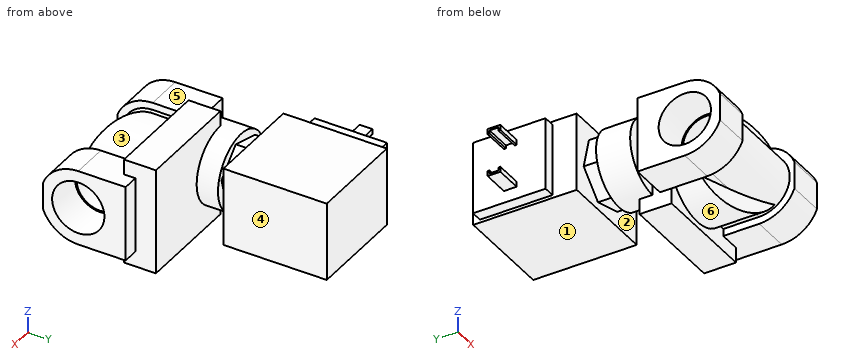
```python
from build123d import *

# Parameters (mm, degrees)
SKETCH1_R                = 18.0086
BOSS_EXTRUDE1_DEPTH      = 20.9296
CUT_EXTRUDE1_DEPTH       = 19.0086
CUT_EXTRUDE1_DEPTH_BACK  = 19.0086
BOSS_EXTRUDE2_DEPTH      = 16.129
BOSS_EXTRUDE3_DEPTH      = 14.0335
SKETCH6_W                = 40.132
SKETCH6_H                = 40.132
BOSS_EXTRUDE4_DEPTH      = 12.0777
SKETCH7_R                = 14.2875
BOSS_EXTRUDE5_DEPTH      = 8.0772
BOSS_EXTRUDE5_DEPTH_BACK = 4.826
BOSS_EXTRUDE6_DEPTH      = 5.9817
SKETCH11_W               = 41.656
SKETCH11_H               = 29.718
BOSS_EXTRUDE7_DEPTH      = 39.116
SKETCH12_W               = 29.718
SKETCH12_H               = 39.116
SKETCH12_W_2             = 27.432
SKETCH12_H_2             = 27.432
CUT_EXTRUDE2_DEPTH       = 4.318
BOSS_EXTRUDE8_DEPTH      = 10.16


with BuildPart() as part:
    # Sketch1 → Boss-Extrude1 (new body)
    with BuildSketch(Plane(origin=(0, 0, 0), x_dir=(1, 0, 0), z_dir=(0, 1, 0))):
        Circle(SKETCH1_R)
    extrude(amount=-BOSS_EXTRUDE1_DEPTH)

    # Sketch2 → Cut-Extrude1 (cut, two sides)
    with BuildSketch(Plane.XY) as cut_extrude1_sk:
        Polygon((-18.0086, -8.382), (18.0086, -20.9296), (-18.0086, -20.9296), align=None)
    extrude(amount=CUT_EXTRUDE1_DEPTH, mode=Mode.SUBTRACT)
    extrude(cut_extrude1_sk.sketch, amount=-CUT_EXTRUDE1_DEPTH_BACK, mode=Mode.SUBTRACT)

    # Sketch3 → Boss-Extrude2 (add, symmetric)
    with BuildSketch(Plane(origin=(0, 0, 0), x_dir=(0, 0, -1), z_dir=(1, 0, 0))):
        with BuildLine():
            Line((-11.557, 0), (-11.557, -13.589))
            ThreePointArc((-11.557, -13.589), (0, -25.146), (11.557, -13.589))
            Line((11.557, -13.589), (11.557, 0))
            Line((11.557, 0), (-11.557, 0))
        make_face()
    extrude(amount=BOSS_EXTRUDE2_DEPTH, both=True)

    # Sketch5 → Boss-Extrude3 (add)
    with BuildSketch(Plane.ZY.offset(16.129)):
        with BuildLine():
            Line((-14.2875, 4.318), (-14.2875, -13.589))
            ThreePointArc((-14.2875, -13.589), (-11.777489603, -21.677472965), (-5.129369479, -26.924))
            Line((-5.129369479, -26.924), (5.129369479, -26.924))
            ThreePointArc((5.129369479, -26.924), (11.777489603, -21.677472965), (14.2875, -13.589))
            Line((14.2875, -13.589), (14.2875, 4.318))
            Line((14.2875, 4.318), (-14.2875, 4.318))
        make_face()
    boss_extrude3 = extrude(amount=BOSS_EXTRUDE3_DEPTH)

    # Mirror1: Boss-Extrude3 across plane
    add(boss_extrude3.mirror(Plane(origin=(0, 0, 0), x_dir=(0, 0, 1), z_dir=(1, 0, 0))))

    # Sketch6 → Boss-Extrude4 (add)
    with BuildSketch(Plane(origin=(0, 0, 0), x_dir=(1, 0, 0), z_dir=(0, 1, 0))):
        with Locations((4.0005, 0)):
            Rectangle(SKETCH6_W, SKETCH6_H)
    extrude(amount=BOSS_EXTRUDE4_DEPTH)

    # Sketch7 → Boss-Extrude5 (add, two sides)
    with BuildSketch(Plane(origin=(0, 12.0777, 0), x_dir=(1, 0, 0), z_dir=(0, 1, 0))) as boss_extrude5_sk:
        with Locations((-15.56738583, 0)):
            Circle(SKETCH7_R)
    extrude(amount=BOSS_EXTRUDE5_DEPTH)
    extrude(boss_extrude5_sk.sketch, amount=-BOSS_EXTRUDE5_DEPTH_BACK)

    # Sketch8 → 1/2 NPT Tapped Hole1 (revolve, cut)
    with BuildSketch(Plane(origin=(30.1625, -13.589, 0), x_dir=(0, 0, -1), z_dir=(0, 1, 0))):
        Polygon((0, 0), (0, 28.003563693), (8.9281, 22.63902), (8.9281, 13.57122), (9.479720499, 13.57122), (9.886061, 0), align=None)
    f_1_2_npt_tapped_hole1 = revolve(axis=Axis((36.5125, -13.589, 0), (-1, 0, 0)), mode=Mode.SUBTRACT)

    # Mirror2: 1/2 NPT Tapped Hole1 across plane
    add(f_1_2_npt_tapped_hole1.mirror(Plane(origin=(0, 0, 0), x_dir=(0, 0, 1), z_dir=(1, 0, 0))), mode=Mode.SUBTRACT)

    # Sketch10 → Boss-Extrude6 (add)
    with BuildSketch(Plane(origin=(0, 20.1549, 0), x_dir=(1, 0, 0), z_dir=(0, 1, 0))):
        Polygon((-6.716522972, 8.880967834), (-18.833098156, 12.105555998), (-27.683961014, 3.224588164), (-24.418248689, -8.880967834), (-12.301673505, -12.105555998), (-3.450810647, -3.224588164), align=None)
    extrude(amount=BOSS_EXTRUDE6_DEPTH)

    # Sketch11 → Boss-Extrude7 (add)
    with BuildSketch(Plane(origin=(0, 26.1366, 0), x_dir=(1, 0, 0), z_dir=(0, 1, 0))):
        with Locations((-15.56738583, 0)):
            Rectangle(SKETCH11_W, SKETCH11_H)
    extrude(amount=BOSS_EXTRUDE7_DEPTH)

    # Sketch12 → Cut-Extrude2 (cut)
    with BuildSketch(Plane.ZY.offset(36.39538583)):
        with Locations((0, 45.6946)):
            Rectangle(SKETCH12_W, SKETCH12_H)
        with Locations((0, 48.9966)):
            Rectangle(SKETCH12_W_2, SKETCH12_H_2, mode=Mode.SUBTRACT)
    extrude(amount=-CUT_EXTRUDE2_DEPTH, mode=Mode.SUBTRACT)

    # Sketch13 → Boss-Extrude8 (add)
    with BuildSketch(Plane.ZY.offset(36.39538583)):
        Polygon((-7.1882, 51.0286), (-9.144, 51.0286), (-9.144, 46.2026), (-7.1882, 46.2026), (-7.1882, 46.9646), (-8.382, 46.9646), (-8.382, 50.2666), (-7.1882, 50.2666), align=None)
        Polygon((7.1882, 46.9646), (7.1882, 46.2026), (9.144, 46.2026), (9.144, 51.0286), (7.1882, 51.0286), (7.1882, 50.2666), (8.382, 50.2666), (8.382, 46.9646), align=None)
    extrude(amount=BOSS_EXTRUDE8_DEPTH)


solid = part.part
```
Part model, mm, in its own coordinate system. Face numbers are marked on the shaded views. A direction names the side the tool comes from. Give positions to 0.01 mm unless a question says otherwise; leave off trailing zeros. Order: outer loops, then holes, each group sorted by start corner. A loop starts at its lowest first (then second) coordinate and runs counter-clockwise, first axis right, second up. Notation, with made-up numbers: (37.5, -16) - (92.5, -16) arc R14 ccw to (92.5, -7) - close; hole circle Ø1 at (-18.5, 77). An arc over 180 degrees is marked (long way). Use one line per item in the form item = value.
Item 1: Pin check, flat tips, straight feed: pin 1 Ø9.5 at (y, z) = (-11, -0.5) entering from -X; pin 2 Ø23 at (y, z) = (-8, 5) entering from -X; pin 3 Ø0.6 at (x, z) = (-39, 7.5) entering from +Y. Stop position of each tip, or through.
Solution:
pin_1 = -6.6
pin_2 = -30.16
pin_3 = 51.03
Item 2: Two-plate mould, pull along X, no slides. Class the marked faces 4, 5 and 6: released by +X, released by -X, zero draft, split by the parting line, or undercut.
Solution:
face_4 = released by +X
face_5 = zero draft
face_6 = undercut
Item 3: Slice it at C-C on x = -9.5. Give the cut face in (y, z), and give its area (3 significant figures).
Solution:
outline = (-13.59, -11.56) - (-11.35, -11.56) - (-11.35, -15.3) - (0, -15.3) - (0, -20.07) - (12.08, -20.07) - (12.08, -12.94) - (20.15, -12.94) - (20.15, -9.62) - (26.14, -9.62) - (26.14, -14.86) - (65.25, -14.86) - (65.25, 14.86) - (26.14, 14.86) - (26.14, 9.29) - (20.15, 9.29) - (20.15, 12.94) - (12.08, 12.94) - (12.08, 20.07) - (0, 20.07) - (0, 15.3) - (-11.35, 15.3) - (-11.35, 11.56) - (-13.59, 11.56) arc R11.56 ccw to start; hole circle Ø17.86 at (-13.59, 0)
area = 2,330 mm2
Item 4: Slice it at B-B on y = 58.5. Give the cut face in (x, z), and give its area (3 significant figures).
Solution:
outline = (-36.4, -13.72) - (-32.08, -13.72) - (-32.08, -14.86) - (5.26, -14.86) - (5.26, 14.86) - (-32.08, 14.86) - (-32.08, 13.72) - (-36.4, 13.72) - close
area = 1,230 mm2
Item 5: Probe probe 1 along Y at (x, z) = (13.5, 0); probe 2 along Y at (x, z) = (-10.75, 0); probe 3 along Y at (x, z) = (-19, -7). List the from-to ranges inside material, lowest first. Write a range as from..to.
Solution:
probe_1 = -25.15..-22.52, -4.66..12.08
probe_2 = -25.15..-22.52, -4.66..65.25
probe_3 = -26.04..-20.09, -7.09..4.32, 7.25..65.25
Item 6: Which spindle directions (+Z, -Z, +X, -X, +Y, -Y) get a long thin tool onto all of the face, cutting with end or side? Do the marked faces 1, 2 and 3. Say none if no direction does.
Solution:
face_1 = -Z, +X, -X, +Y
face_2 = none
face_3 = +Z, -Y
Item 7: Slice it at D-D on y = 22.5. Give the cut face in (x, z).
Solution:
outline = (-27.68, -3.22) - (-18.83, -12.11) - (-6.72, -8.88) - (-3.45, 3.22) - (-12.3, 12.11) - (-24.42, 8.88) - close
Item 8: Slice it at A-A on x = -26. Give the cut face in (y, z) (1 decimal).
Solution:
outline = (-26.9, -5.1) arc R14.3 ccw to (-13.6, -14.3) - (4.3, -14.3) - (4.3, 14.3) - (-13.6, 14.3) arc R14.3 ccw to (-26.9, 5.1) - close; (7.3, -9.8) - (20.2, -9.8) - (20.2, -4.9) - (26.1, -4.9) - (26.1, -14.9) - (65.3, -14.9) - (65.3, 14.9) - (26.1, 14.9) - (26.1, 3) - (20.2, 3) - (20.2, 9.8) - (7.3, 9.8) - close; hole circle Ø19.5 at (-13.6, 0)
